Autodesk Fusion 360 part; units mm, degrees
sketch "Esquisse1" plane through (0, 0, 0) normal (0, 0, 1) x (1, 0, 0)
  line L0 (0.4, 40) -> (70, 40)
  line L1 (70, 40) -> (70, 20.4)
  line L2 (70, 20.4) -> (0.4, 20.4)
  line L3 (0.4, 20.4) -> (0.4, 40)
  dimension "d1" = 69.6
  dimension "d2" = 19.6
extrude "Extrusion1" add sketch "Esquisse1" along normal blind 3
sketch "Esquisse2" plane through (0, 0, 0) normal (0, 0, -1) x (1, 0, 0)
  line L0 (70, -20.4) -> (0.4, -20.4)
  line L1 (0.4, -20.4) -> (0.4, -40)
  line L2 (0.4, -40) -> (70, -40)
  line L3 (70, -40) -> (70, -20.4)
  line L4 (7.6, -22.3) -> (12.8, -22.3)
  line L5 (12.8, -22.3) -> (12.8, -24.5)
  line L6 (12.8, -24.5) -> (7.6, -24.5)
  line L7 (7.6, -24.5) -> (7.6, -22.3)
  line L8 (10.2, -22.3) -> (10.2, -24.5) construction
  line L9 (35.2, -20.4) -> (35.2, -40) construction
  line L10 (57.6, -22.3) -> (57.6, -24.5)
  line L11 (62.8, -22.3) -> (57.6, -22.3)
  line L12 (62.8, -24.5) -> (62.8, -22.3)
  line L13 (57.6, -24.5) -> (62.8, -24.5)
  line L14 (0.4, -30.2) -> (70, -30.2) construction
  line L15 (7.6, -38.1) -> (12.8, -38.1)
  line L16 (12.8, -38.1) -> (12.8, -35.9)
  line L17 (12.8, -35.9) -> (7.6, -35.9)
  line L18 (7.6, -35.9) -> (7.6, -38.1)
  line L19 (62.8, -38.1) -> (57.6, -38.1)
  line L20 (62.8, -35.9) -> (62.8, -38.1)
  line L21 (57.6, -35.9) -> (62.8, -35.9)
  line L22 (57.6, -38.1) -> (57.6, -35.9)
  dimension "d5" = 25
  dimension "d12" = 5.2
  dimension "d13" = 2.2
  dimension "d14" = 1.9
extrude "Extrusion2" cut sketch "Esquisse2" against normal blind 2 contours L4 L5 L6 L7 | L10 L11 L12 L13 | L15 L16 L17 L18 | L19 L20 L21 L22
sketch "Esquisse3" plane through (0, 0, 3) normal (0, 0, 1) x (-1, 0, 0)
  line L0 (-0.4, -20.4) -> (-70, -20.4)
  line L1 (-70, -20.4) -> (-70, -40)
  line L2 (-70, -40) -> (-0.4, -40)
  line L3 (-0.4, -40) -> (-0.4, -20.4)
  line L4 (-22.45, -37.9) -> (-47.95, -37.9)
  line L5 (-47.95, -37.9) -> (-47.95, -22.5)
  line L6 (-47.95, -22.5) -> (-22.45, -22.5)
  line L7 (-22.45, -22.5) -> (-22.45, -37.9)
  line L8 (-0.4, -30.2) -> (-70, -30.2) construction
  line L9 (-35.2, -40) -> (-35.2, -20.4) construction
  dimension "d8" = 25.5
  dimension "d9" = 15.4
extrude "Extrusion3" cut sketch "Esquisse3" against normal blind 2 contours L4 L5 L6 L7
sketch "Esquisse4" plane through (0, 0, 1) normal (0, 0, 1) x (-1, 0, 0)
  line L0 (-22.45, -22.5) -> (-47.95, -22.5)
  line L1 (-47.95, -22.5) -> (-47.95, -37.9)
  line L2 (-47.95, -37.9) -> (-22.45, -37.9)
  line L3 (-22.45, -37.9) -> (-22.45, -22.5)
  line L4 (-22.45, -22.5) -> (-25.45, -22.5)
  line L5 (-25.45, -22.5) -> (-25.45, -37.9)
  line L6 (-25.45, -37.9) -> (-22.45, -37.9)
  line L7 (-22.45, -37.9) -> (-22.45, -22.5)
  dimension "d15" = 3
extrude "Extrusion4" cut sketch "Esquisse4" against normal blind 3 contours L0 L2 L3 L4 L5 L6 L7
sketch "Esquisse5" plane through (0, 40, 0) normal (0, 1, 0) x (-1, 0, 0)
  line L0 (-70, 0) -> (-0.4, 0)
  line L1 (-0.4, 0) -> (-0.4, 3)
  line L2 (-0.4, 3) -> (-70, 3)
  line L3 (-70, 3) -> (-70, 0)
  line L4 (-35.2, 3) -> (-35.2, 0) construction
  line L5 (-42.7, 3) -> (-27.7, 3)
  line L6 (-27.7, 3) -> (-27.7, 1)
  line L7 (-27.7, 1) -> (-42.7, 1)
  line L8 (-42.7, 1) -> (-42.7, 3)
  dimension "d18" = 15
  dimension "d19" = 2
extrude "Extrusion5" cut sketch "Esquisse5" against normal blind 21 contours L2 L5 L6 L7 L8
sketch "Esquisse6" plane through (0, 0, 3) normal (0, 0, 1) x (-1, 0, 0)
  line L0 (-42.7, -22.5) -> (-42.7, -20.4)
  line L1 (-42.7, -20.4) -> (-70, -20.4)
  line L2 (-70, -20.4) -> (-70, -40)
  line L3 (-70, -40) -> (-42.7, -40)
  line L4 (-42.7, -40) -> (-42.7, -37.9)
  line L5 (-42.7, -37.9) -> (-47.95, -37.9)
  line L6 (-47.95, -37.9) -> (-47.95, -22.5)
  line L7 (-47.95, -22.5) -> (-42.7, -22.5)
  line L8 (-70, -40) -> (-67.5, -40)
  line L9 (-67.5, -40) -> (-67.5, -20.4)
  line L10 (-67.5, -20.4) -> (-70, -20.4)
  line L11 (-70, -20.4) -> (-70, -40)
  line L12 (-35.2, -39) -> (-35.2, -18) construction
  line L13 (-0.4, -20.4) -> (-0.4, -40)
  line L14 (-2.9, -20.4) -> (-0.4, -20.4)
  line L15 (-2.9, -40) -> (-2.9, -20.4)
  line L16 (-0.4, -40) -> (-2.9, -40)
  dimension "d22" = 2.5
  dimension "d23" = 34.8
extrude "Extrusion6" cut sketch "Esquisse6" against normal blind 2 contours L1 L2 L3 L8 L9 L10 L11 | L13 L14 L15 L16
For this review, take the finished solid that the model builds, in its own axes (mm). A direction names the side the tool comes from. Coordinates: 2 decimals unless noted, no trailing zeros. Order: outer loops, then holes, each group sorted by start corner. A loop starts at its lowest first (then second) coordinate and runs counter-clockwise, first axis right, second up. Notation, with made-up numbers: (52, 87) - (75, 87) arc R31 ccw to (75, 113) - close; hole circle Ø7 at (-26.5, -37). An arc over 180 degrees is marked (long way). Answer as a JSON object with one key per item and string values. Group by question number.
1. For probe 1 along X at (y, z) = (23, 0.65); probe 2 along X at (y, z) = (22.75, 1.1); probe 3 along Y at (x, z) = (9, 0.6), list the stretches that pass through material, from the lowest coordinate up.
2. Clearance check with flat-ended pins moving along their axes: P1, Ø1.6, axis at y = 21.5, z = 2, coming from the -X side; P2, Ø1.1, axis at x = 9.5, y = 23.5, coming from the -Z side. State where each tip first meets the part, or that it passes through.
3. We need section D-D on y = 27.75. State the section outline as (x, z) points.
4. We need section C-C on x = 61. State the section outline as (y, z) points.
5. We need section A-A on y = 37. State the section outline as (x, z) points, then the cut area to 3 significant figures.
6. We need section B-B on y = 21.5. State the section outline as (x, z) points.
7. For faces 1 (the flat face through (60, 38.1, 1)), 2 (the flat face through (47.95, 30, 2)), 3 (the flat face through (42.7, 21, 2)), list the 3-axis set-ups (+Z, -Z, +X, -X, +Y, -Y) from which the entire face can be reached by the end or side of a thin tool; tool diameter is ignored.
8. The part is to be moulded in two halves that separate along Y. For faces 4 (the flat face through (60, 22.3, 1)), 5 (the flat face through (67.5, 30, 2)), 6 (the flat face through (34.7, 40, 0.8)), say which applies: pulls with the +Y half, pulls with the -Y half, needs draft (parallel to the pull), parting line crosses it, or undercut.
Final values:
{
 "1": {"probe 1": "0.4 to 7.6, 12.8 to 22.45, 25.45 to 57.6, 62.8 to 70", "probe 2": "2.9 to 7.6, 12.8 to 22.45, 47.95 to 57.6, 62.8 to 67.5", "probe 3": "20.4 to 22.3, 24.5 to 35.9, 38.1 to 40"},
 "2": {"P1": "x = 2.9", "P2": "z = 2"},
 "3": {"outline": "(0.4, 0) - (22.45, 0) - (22.45, 3) - (2.9, 3) - (2.9, 1) - (0.4, 1) - close; (25.45, 0) - (70, 0) - (70, 1) - (67.5, 1) - (67.5, 3) - (47.95, 3) - (47.95, 1) - (25.45, 1) - close"},
 "4": {"outline": "(20.4, 0) - (22.3, 0) - (22.3, 2) - (24.5, 2) - (24.5, 0) - (35.9, 0) - (35.9, 2) - (38.1, 2) - (38.1, 0) - (40, 0) - (40, 3) - (20.4, 3) - close"},
 "5": {"outline": "(0.4, 0) - (7.6, 0) - (7.6, 2) - (12.8, 2) - (12.8, 0) - (22.45, 0) - (22.45, 3) - (2.9, 3) - (2.9, 1) - (0.4, 1) - close; (25.45, 0) - (57.6, 0) - (57.6, 2) - (62.8, 2) - (62.8, 0) - (70, 0) - (70, 1) - (67.5, 1) - (67.5, 3) - (47.95, 3) - (47.95, 1) - (25.45, 1) - close", "area": "124 mm²"},
 "6": {"outline": "(0.4, 0) - (70, 0) - (70, 1) - (67.5, 1) - (67.5, 3) - (42.7, 3) - (42.7, 1) - (27.7, 1) - (27.7, 3) - (2.9, 3) - (2.9, 1) - (0.4, 1) - close"},
 "7": {"face 1": "-Z", "face 2": "+Z", "face 3": "+Z, +Y, -Y"},
 "8": {"face 4": "undercut", "face 5": "needs draft", "face 6": "pulls with the +Y half"}
}
